from build123d import *

# Parameters (mm, degrees)
SKETCH_1_R          = 4.5
EXTRUDE_1_DEPTH     = 2
SKETCH_2_R          = 2.5
SKETCH_2_R_2        = 2
EXTRUDE_2_DEPTH     = 12
FILLET_1_R          = 1
CHAMFER_1_SIZE      = 0.5
CUT_EXTRUDE_1_DEPTH = 1


with BuildPart() as part:
    # 草图1 → 凸台-拉伸1 (new body)
    with BuildSketch(Plane.XY):
        Circle(SKETCH_1_R)
    extrude(amount=EXTRUDE_1_DEPTH)

    # 草图2 → 凸台-拉伸2 (add)
    with BuildSketch(Plane.XY.offset(2)):
        Circle(SKETCH_2_R)
        Circle(SKETCH_2_R_2, mode=Mode.SUBTRACT)
    extrude(amount=EXTRUDE_2_DEPTH)

    # 圆角1
    fillet_1_edges = [part.edges().sort_by_distance(p)[0] for p in [
        (-4.5, 0, 0),
    ]]
    fillet(fillet_1_edges, radius=FILLET_1_R)

    # 倒角1
    chamfer_1_edges = [part.edges().sort_by_distance(p)[0] for p in [
        (-4.5, 0, 2),
    ]]
    chamfer(chamfer_1_edges, length=CHAMFER_1_SIZE)

    # 草图3 → 切除-拉伸1 (cut)
    with BuildSketch(Plane(origin=(0, 0, 0), x_dir=(-1, 0, 0), z_dir=(0, 0, -1))):
        Polygon((0.866025404, -1.5), (1.732050808, 0), (0.866025404, 1.5), (-0.866025404, 1.5), (-1.732050808, 0), (-0.866025404, -1.5), align=None)
    extrude(amount=-CUT_EXTRUDE_1_DEPTH, mode=Mode.SUBTRACT)


solid = part.part
Input: part model. Units: mm. Frame: model coordinates. A direction names the side the tool comes from. Coordinates: 2 decimals unless noted, no trailing zeros. Loops run counter-clockwise (first coordinate to the right, second up) from the corner with the lowest first, then second, coordinate; pieces in that order, holes last. Notation, with made-up numbers: (31.5, 40) -> (50.5, 40) arc R16 cw to (50.5, 51) -> close; hole circle Ø11 at (28.25, 14). An arc over 180 degrees is marked (long way). One line per item, written item: value.
(1) Cut plane A-A (z = 2.5). Output: boundary loops of the cut face in (x, y).
Answer below:
outline: circle Ø5 at (0, 0); hole circle Ø4 at (0, 0)
(2) Ray query, line 1 along Y through (x, z) = (0, 6.25); line 2 along Z through (x, y) = (-3, -1.5); line 3 along Y through (x, z) = (1.5, 7.75). Return the intervals inside material, ascending.
Answer below:
line 1: y = -2.5 to -2, 2 to 2.5
line 2: z = 0 to 2
line 3: y = -2 to -1.32, 1.32 to 2
(3) Cut plane B-B (x = 0). Output: boundary loops of the cut face in (y, z), then the cut area to 3 significant figures.
Answer below:
outline: (-4.5, 1) arc R1 ccw to (-3.5, 0) -> (-1.5, 0) -> (-1.5, 1) -> (1.5, 1) -> (1.5, 0) -> (3.5, 0) arc R1 ccw to (4.5, 1) -> (4.5, 1.5) -> (4, 2) -> (2.5, 2) -> (2.5, 14) -> (2, 14) -> (2, 2) -> (-2, 2) -> (-2, 14) -> (-2.5, 14) -> (-2.5, 2) -> (-4, 2) -> (-4.5, 1.5) -> close
area: 26.3 mm2
(4) Set-up query: faces 5 (the face through (-0.54, -2.44, 7.92)), 6 (the face through (-1, 2, 14)), 7 (the face through (-1.293, -0.76, 0.493)). Return all of +Z, -Z, +X, -X, +Y, -Y with unobstructed straight access to the full face (end or side cutting, diameter ignored); none if empty.
Answer below:
face 5: +Z
face 6: +Z, +X, -X, +Y, -Y
face 7: -Z
(5) Pin query (flat end, axial travel): pin 1 Ø1.2 at (x, y) = (-0.5, 0.5) entering from +Z; pin 2 Ø0.5 at (x, z) = (0, 0.5) entering from +Y; pin 3 Ø1.5 at (y, z) = (1.5, 2) entering from -X; pin 4 Ø1 at (x, y) = (2, 2.5) entering from -Z. Return the tip coordinate at first contact, or that it passes through.
Answer below:
pin 1: stops at z = 2
pin 2: stops at y = 4.47
pin 3: stops at x = -4.4
pin 4: stops at z = 0
(6) Draft query along X for faces 1 (the face through (0, 0, 2)), 2 (the face through (0, -1.5, 0.5)), 3 (the face through (-2, -2, 2)), 4 (the face through (-0.59, 4.46, 1.25)). Return one class per face: pulls with the +X half, pulls with the -X half, needs draft (parallel to the pull), parting line crosses it, or undercut.
Answer below:
face 1: undercut
face 2: undercut
face 3: needs draft
face 4: parting line crosses it
